```python
from build123d import *

# Parameters (mm, degrees)
F0_W     = 88.9
F0_H     = 25.4
F1_DEPTH = 508
F3_DEPTH = 12.7
F4_W     = 44.45
F4_H     = 44.45
F5_DEPTH = 4.445
F6_DEPTH = 7.62
F8_R     = 21.5773
F9_DEPTH = 20.32


with BuildPart() as f1:
    # F0 (on Front) → F1 (new body)
    with BuildSketch(Plane.XZ):
        with Locations((-4.590311, -8.587727)):
            Rectangle(F0_W, F0_H)
    extrude(amount=F1_DEPTH)

    # F2 (on face) → F3 (join)
    with BuildSketch(Plane(origin=(0, 0, -21.287727), x_dir=(1, 0, 0), z_dir=(0, 0, -1))):
        Polygon((-4.590311, 88.9), (-49.040311, 88.9), (-49.040311, 0), (39.859689, 0), (39.859689, 88.9), align=None)
        Polygon((-49.040311, 508), (-49.040311, 419.1), (-4.590311, 419.1), (39.859689, 419.1), (39.859689, 508), align=None)
    extrude(amount=F3_DEPTH)

    # F4 (on face) → F5 (join)
    with BuildSketch(Plane(origin=(0, 0, -21.287727), x_dir=(1, 0, 0), z_dir=(0, 0, -1))):
        with Locations((17.634689, 231.775)):
            Rectangle(F4_W, F4_H)
        Polygon((-49.040311, 209.55), (-4.590311, 209.55), (-4.590311, 254), (-4.590311, 298.45), (-49.040311, 298.45), align=None)
        with Locations((17.634689, 276.225)):
            Rectangle(F4_W, F4_H)
    extrude(amount=F5_DEPTH)

    # F4 (on face) → F6 (join)
    with BuildSketch(Plane(origin=(0, 0, -21.287727), x_dir=(1, 0, 0), z_dir=(0, 0, -1))):
        with Locations((17.634689, 231.775)):
            Rectangle(F4_W, F4_H)
        Polygon((-49.040311, 209.55), (-4.590311, 209.55), (-4.590311, 254), (-4.590311, 298.45), (-49.040311, 298.45), align=None)
        with Locations((17.634689, 276.225)):
            Rectangle(F4_W, F4_H)
    extrude(amount=F6_DEPTH)

    # F8 (on face) → F9 (cut)
    with BuildSketch(Plane.XY.offset(4.112273)):
        with Locations((-4.588948, -254.004985)):
            Circle(F8_R)
    extrude(amount=-F9_DEPTH, mode=Mode.SUBTRACT)


solid = f1.part
```
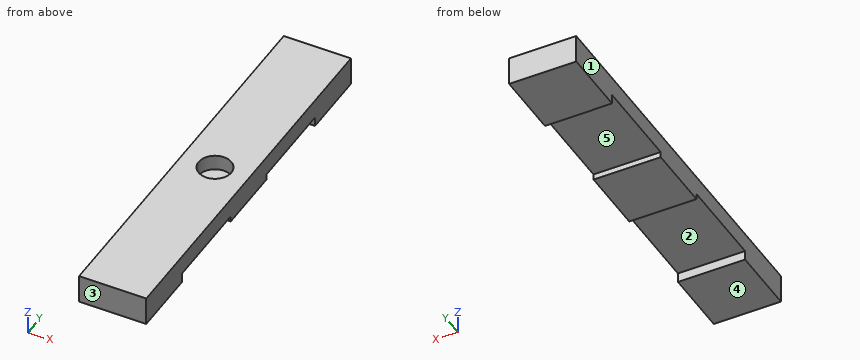
Design review of the part built by this model. Coordinates are the model's own, in mm. Face numbers are marked on the shaded views. A direction names the side the tool comes from. Coordinates: 2 decimals unless noted, no trailing zeros. Order: outer loops, then holes, each group sorted by start corner. A loop starts at its lowest first (then second) coordinate and runs counter-clockwise, first axis right, second up.
1) Take a section at C-C, the plane y = -239.5. Give the boundary of the cut face in (x, z), and give its area (3 significant figures).
2) Mouldability with a two-part tool opening along Y and no side actions: class the marked faces 3, 4 and 5 as +Y half, -Y half, draft (parallel to the pull), parting line (faces both ways), or undercut.
3) Take a section at D-D, the plane x = -4. Give the boundary of the cut face in (y, z).
4) Take a section at A-A, the plane x = -31.5. Give the boundary of the cut face in (y, z), and give its area (3 significant figures).
5) Wall thickness on line 1 along Y through (x, z) = (27, -21.5); line 2 along Y through (x, z) = (-5, -30.5): over which ranges is each line inside the solid? List them lowest first.
6) Clearance check with a flat-ended pin moving along its axis: pin 1 (2 mm diameter, centred on x = -34, y = -94.5, fed in from -Z). State where the tip first meets the part, or that it passes through.
7) Take a section at B-B, the plane z = -7. Give the boundary of the cut face in (x, y), and give its area (3 significant figures).
8) For the marked faces 1 and 2, list the 3-axis set-ups (+Z, -Z, +X, -X, +Y, -Y) from which the entire face can be reached by the end or side of a thin tool; tool diameter is ignored.
Returned:
1. outline: (-49.04, -28.91) - (39.86, -28.91) - (39.86, 4.11) - (11.39, 4.11) - (11.39, -16.21) - (-20.56, -16.21) - (-20.56, 4.11) - (-49.04, 4.11) - close
1. area: 2,290 mm2
2. face 3: -Y half
2. face 4: draft
2. face 5: undercut
3. outline: (-508, -33.99) - (-419.1, -33.99) - (-419.1, -21.29) - (-298.45, -21.29) - (-298.45, -28.91) - (-209.55, -28.91) - (-209.55, -21.29) - (-88.9, -21.29) - (-88.9, -33.99) - (0, -33.99) - (0, 4.11) - (-232.44, 4.11) - (-232.44, -16.21) - (-275.57, -16.21) - (-275.57, 4.11) - (-508, 4.11) - close
4. outline: (-508, -33.99) - (-419.1, -33.99) - (-419.1, -21.29) - (-298.45, -21.29) - (-298.45, -28.91) - (-209.55, -28.91) - (-209.55, -21.29) - (-88.9, -21.29) - (-88.9, -33.99) - (0, -33.99) - (0, 4.11) - (-508, 4.11) - close
4. area: 15,800 mm2
5. line 1: y = -508 to -419.1, -298.45 to -209.55, -88.9 to 0
5. line 2: y = -508 to -419.1, -88.9 to 0
6. pin 1: stops at z = -21.29
7. outline: (-49.04, -508) - (39.86, -508) - (39.86, 0) - (-49.04, 0) - close; hole circle Ø43.15 at (-4.59, -254)
7. area: 43,700 mm2
8. face 1: +Z, -Z, -X, +Y, -Y
8. face 2: -Z, +X, -X
